```python
from build123d import *

# Parameters (mm, degrees)
F1_DEPTH  = 23
F4_D      = 6
F5_D      = 6
F6_W      = 75
F6_H      = 5.3172297776
F7_DEPTH  = 8
F8_SIZE2  = 37.5
F8_SIZE   = 8
F9_SIZE2  = 37.5
F9_SIZE   = 8
F10_SIZE2 = 37.49999
F10_SIZE  = 7.99999
F11_SIZE2 = 37.49999
F11_SIZE  = 7.99999
F12_R     = 8.65
F13_DEPTH = 4


# Not quite as in the source:
# - a fillet or chamfer is up to 0.001 mm smaller than in the source, because OpenCascade refuses the exact size


with BuildPart() as f1:
    # F0 (on Top) → F1 (new body)
    with BuildSketch(Plane.XY):
        with BuildLine():
            Line((37.5, 20), (-37.5, 20))
            Line((-37.5, 20), (-37.5, 0))
            Line((-37.5, 0), (-14.1, 0))
            ThreePointArc((-14.1, 0), (0, 14.1), (14.1, 0))
            Line((14.1, 0), (37.5, 0))
            Line((37.5, 0), (37.5, 20))
        make_face()
    extrude(amount=F1_DEPTH)

    # F4 (through all)
    with Locations(Plane.XZ):
        with Locations((-25.8, 11.5)):
            Hole(F4_D / 2)

    # F5 (through all)
    with Locations(Plane.XZ):
        with Locations((25.8, 11.5)):
            Hole(F5_D / 2)

    # F6 (on face) → F7 (join)
    with BuildSketch(Plane(origin=(0, 20, 0), x_dir=(-1, 0, 0), z_dir=(0, 1, 0))):
        with Locations((0, 20.3413851112)):
            Rectangle(F6_W, F6_H)
        with Locations((0, 2.6586148888)):
            Rectangle(F6_W, F6_H)
    extrude(amount=F7_DEPTH)

    # F8
    f8_edges = [f1.edges().sort_by_distance(p)[0] for p in [
        (37.5, 28, 2.658615),
    ]]
    f8_side = f1.faces().sort_by_distance((37.5, 12.185127, 11.5))[0]
    chamfer(f8_edges, length=F8_SIZE, length2=F8_SIZE2, reference=f8_side)

    # F9
    f9_edges = [f1.edges().sort_by_distance(p)[0] for p in [
        (37.5, 28, 20.341385),
    ]]
    f9_side = f1.faces().sort_by_distance((37.5, 11.185045, 12.248388))[0]
    chamfer(f9_edges, length=F9_SIZE, length2=F9_SIZE2, reference=f9_side)

    # F10 (size 8 and 37.5 in the source; OpenCascade refuses exactly that, so slightly less here)
    f10_edges = [f1.edges().sort_by_distance(p)[0] for p in [
        (-37.5, 28, 20.341385),
    ]]
    f10_side = f1.faces().sort_by_distance((-37.5, 12.185127, 11.5))[0]
    chamfer(f10_edges, length=F10_SIZE, length2=F10_SIZE2, reference=f10_side)

    # F11 (size 8 and 37.5 in the source; OpenCascade refuses exactly that, so slightly less here)
    f11_edges = [f1.edges().sort_by_distance(p)[0] for p in [
        (-37.5, 28, 2.658615),
    ]]
    f11_side = f1.faces().sort_by_distance((-37.5, 11.185046, 10.751613))[0]
    chamfer(f11_edges, length=F11_SIZE, length2=F11_SIZE2, reference=f11_side)

    # F12 (on face) → F13 (cut, symmetric)
    with BuildSketch(Plane(origin=(0, 20, 0), x_dir=(-1, 0, 0), z_dir=(0, 1, 0))):
        with Locations((25.8, 11.5)):
            Circle(F12_R)
        with Locations((-25.8, 11.5)):
            Circle(F12_R)
    extrude(amount=F13_DEPTH, both=True, mode=Mode.SUBTRACT)


solid = f1.part
```
Model file for the job. Use its own axes, mm. A direction names the side the tool comes from. Coordinates: 2 decimals unless noted, no trailing zeros. Loops run counter-clockwise (first coordinate to the right, second up) from the corner with the lowest first, then second, coordinate; pieces in that order, holes last. Notation, with made-up numbers: (34.5, 30) - (53.5, 30) arc R21 ccw to (53.5, 38) - close; hole circle Ø4 at (12.25, 47). An arc over 180 degrees is marked (long way). Answer as a JSON object with one key per item and string values. Group by question number.
(1) Cut at D-D (x = -1.5). Give the cut face in (y, z), then the cut area to 3 significant figures.
(2) Flat gauge pins, fed straight in: pin 1 (4.5 mm diameter, centred on x = 34.5, z = 10.5, fed in from +Y); pin 2 (5 mm diameter, centred on x = -27, z = 8, fed in from +Y); pin 3 (6.5 mm diameter, centred on x = 7, y = 24, fed in from -Z); pin 4 (1.5 mm diameter, centred on x = 24, z = 20.5, fed in from +Y). Where does each tip first touch, or does it go through?
(3) Tool access for faces 5 (the face through (28.8, 8.1, 11.6)), 6 (the face through (-30, 16, 12)), 7 (the face through (35, 20, 11)): list every direction of +Z, -Z, +X, -X, +Y, -Y with a clear straight run to the whole face (end or side of a thin tool).
(4) Two-plate mould, pull along Z, no slides. Class faces 1 (the face through (1, 17, 23)), 2 (the face through (0, 23, 17.683)), 3 (the face through (0, 23, 5.317)), 4 (the face through (37.5, 10, 11)): released by +Z, released by -Z, zero draft, split by the parting line, or undercut.
(5) Probe line 1 along Z through (x, y) = (11.5, 25); line 2 along Z through (x, y) = (25.8, 13.25); line 3 along X through (y, z) = (18.5, 11.25). List the from-to ranges inside material, lowest first.
(6) Cut at C-C (x = -25.8). Give the cut face in (y, z), then the cut area to 3 significant figures.
(7) Cut at A-A (y = 9.75). Give the cut face in (x, z), then the cut area to 3 significant figures.
(8) Cut at B-B (z = 11.5). Give the cut face in (x, y), then the cut area to 3 significant figures.
Geometry says:
{
 "1": {"outline": "(14.02, 0) - (27.68, 0) - (27.68, 5.32) - (20, 5.32) - (20, 17.68) - (27.68, 17.68) - (27.68, 23) - (14.02, 23) - close", "area": "219 mm^2"},
 "2": {"pin 1": "stops at y = 20", "pin 2": "stops at y = 16", "pin 3": "stops at z = 0", "pin 4": "stops at y = 23.04"},
 "3": {"face 5": "+Y, -Y", "face 6": "+Y", "face 7": "+X, -X, +Y"},
 "4": {"face 1": "released by +Z", "face 2": "undercut", "face 3": "undercut", "face 4": "zero draft"},
 "5": {"line 1": "z = 0 to 5.32, 17.68 to 23", "line 2": "z = 0 to 8.5, 14.5 to 23", "line 3": "x = -37.5 to -34.45, -17.15 to 17.15, 34.45 to 37.5"},
 "6": {"outline": "(0, 0) - (22.5, 0) - (22.5, 2.85) - (16, 2.85) - (16, 8.5) - (0, 8.5) - close; (0, 14.5) - (16, 14.5) - (16, 20.15) - (22.5, 20.15) - (22.5, 23) - (0, 23) - close", "area": "309 mm^2"},
 "7": {"outline": "(-37.5, 0) - (-10.19, 0) - (-10.19, 23) - (-37.5, 23) - close; (10.19, 0) - (37.5, 0) - (37.5, 23) - (10.19, 23) - close; hole circle Ø6 at (-25.8, 11.5); hole circle Ø6 at (25.8, 11.5)", "area": "1,200 mm^2"},
 "8": {"outline": "(-37.5, 0) - (-28.8, 0) - (-28.8, 16) - (-34.45, 16) - (-34.45, 20) - (-37.5, 20) - close; (-22.8, 0) - (-14.1, 0) arc R14.1 cw to (14.1, 0) - (22.8, 0) - (22.8, 16) - (17.15, 16) - (17.15, 20) - (-17.15, 20) - (-17.15, 16) - (-22.8, 16) - close; (28.8, 0) - (37.5, 0) - (37.5, 20) - (34.45, 20) - (34.45, 16) - (28.8, 16) - close", "area": "857 mm^2"}
}
